```python
from build123d import *

# Parameters (mm, degrees)
F0_R     = 7.9375
F1_DEPTH = 3.175


with BuildPart() as f1:
    # F0 (on Front) → F1 (new body)
    with BuildSketch(Plane.XZ):
        with BuildLine():
            ThreePointArc((18.536816, 5.08), (-8.902928, 25.271378), (-31.75, 0))
            ThreePointArc((-31.75, 0), (0, -31.75), (31.75, 0))
            Line((31.75, 0), (24.75852, 0))
            ThreePointArc((24.75852, 0), (20.742427, 1.431311), (18.536816, 5.08))
        make_face()
        with Locations((-2.4638, -4.0894)):
            Circle(F0_R, mode=Mode.SUBTRACT)
    extrude(amount=F1_DEPTH)


solid = f1.part
```
Verification items for the finished model (mm, model axes). A direction names the side the tool comes from. Give positions to 0.01 mm unless a question says otherwise; leave off trailing zeros. Order: outer loops, then holes, each group sorted by start corner. A loop starts at its lowest first (then second) coordinate and runs counter-clockwise, first axis right, second up. Notation, with made-up numbers: M -1,81.25 L 8,81.25 A14 cw 8,103.25 Z; hole C 18,75 d2. An arc over 180 degrees is marked long. Answer in a Markdown table with one row per item. Add a question column.
Item 1: Scan lines: probe 1 along X at (y, z) = (-0.4, -9); probe 2 along X at (y, z) = (-3, 3); probe 3 along Z at (x, y) = (-7, -1.2). Record each from-to range of solid material in increasing order. Write a range as from..to.
Item 2: Section check A-A, the plane x = 0. Enter the section's corners in (y, z) (3 decimals).
Item 3: Section check D-D, the plane z = 19. Enter the section's corners in (x, y) (3 decimals).
Item 4: Mould release check, pull along Z, two halves, no side actions. Record for faces 1 (the flat face through (-8, 0, 4)), 2 (the cylindrical face through (-10.394, -1.565, -3.74)), 3 (the cylindrical face through (-0.698, -1.565, -31.742)): released by +Z, released by -Z, zero draft, split by the parting line, or undercut.
Item 5: Section check B-B, the plane z = 1. Enter the section's corners in (x, y) (3 decimals), and give its area (3 significant figures).
Item 6: Tool access check on faces 4 (the flat face through (28, -2, 0)), 5 (the cylindrical face through (-8.38, -1.57, 25.32)). Record the directions out of +Z, -Z, +X, -X, +Y, -Y that give a thin tool (end or side, any length) a straight path to the whole face; none if there is none.
Item 7: Gauge pin test, flat ends, axial feed: pin 1 (1.6 mm diameter, centred on x = 28, y = -1.5, fed in from +Z); pin 2 (1.5 mm diameter, centred on x = 1, y = -0.5, fed in from -Z). Record the tip position at first contact, or that the pin passes through.
Filled sheet:
| question | item | result |
|---|---|---|
| 1 | probe 1 | x = -30.45..-8.7, 3.77..30.45 |
| 1 | probe 2 | x = -31.57..-6.03, 1.11..19.36 |
| 1 | probe 3 | z = -30.97..-10.6, 2.42..25.39 |
| 2 | outline | M -3.175,-31.75 L 0,-31.75 L 0,-11.635 L -3.175,-11.635 Z; M -3.175,3.456 L 0,3.456 L 0,24.593 L -3.175,24.593 Z |
| 3 | outline | M -23.207,-3.175 L 10.507,-3.175 L 10.507,0 L -23.207,0 Z |
| 4 | face 1 | zero draft |
| 4 | face 2 | undercut |
| 4 | face 3 | released by -Z |
| 5 | outline | M -31.73,-3.175 L -8.555,-3.175 L -8.555,0 L -31.73,0 Z; M 3.627,-3.175 L 21.338,-3.175 L 21.338,0 L 3.627,0 Z |
| 5 | area | 130 mm^2 |
| 6 | face 4 | +Z, +X, +Y, -Y |
| 6 | face 5 | +Z, +Y, -Y |
| 7 | pin 1 | stops at z = 0 |
| 7 | pin 2 | stops at z = -31.75 |
